Here's how the part is built. I have some questions about the finished solid (model axes, mm). Face numbers are marked on the shaded views. A direction names the side the tool comes from. Round coordinates to 2 decimals unless told otherwise and drop trailing zeros. Loops run counter-clockwise (first coordinate to the right, second up) from the corner with the lowest first, then second, coordinate; pieces in that order, holes last. Notation, with made-up numbers: M -38.5,38 L -31.5,38 A10 cw -31.5,43 Z; hole C 65.25,9.25 d2. An arc over 180 degrees is marked long. Write each question's results on one line, items separated by ' | '. Start each with the question number.
```python
from build123d import *

# Parameters (mm, degrees)
SKETCH1_W           = 40
SKETCH1_H           = 40
BOSS_EXTRUDE1_DEPTH = 10
SKETCH2_R           = 6.5
BOSS_EXTRUDE2_DEPTH = 2
SKETCH3_W           = 7.5
SKETCH3_H           = 20
BOSS_EXTRUDE3_DEPTH = 3
SKETCH4_W           = 6.5
SKETCH4_H           = 1.5
BOSS_EXTRUDE4_DEPTH = 2.5
CUT_EXTRUDE1_DEPTH  = 2.5
CUT_EXTRUDE6_DEPTH  = 12.5
CHAMFER1_SIZE       = 1.5
SKETCH8_W           = 7
SKETCH8_H           = 4
SKETCH8_W_2         = 5
SKETCH8_H_2         = 2
BOSS_EXTRUDE6_DEPTH = 6
SKETCH7_R           = 2.5
SKETCH7_R_2         = 1.5
BOSS_EXTRUDE7_DEPTH = 4.5


with BuildPart() as part:
    # Sketch1 → Boss-Extrude1 (new, symmetric)
    with BuildSketch(Plane.XY):
        Rectangle(SKETCH1_W, SKETCH1_H)
    extrude(amount=BOSS_EXTRUDE1_DEPTH, both=True)

    # Sketch2 → Boss-Extrude2 (add)
    with BuildSketch(Plane(origin=(0, 20, 0), x_dir=(1, 0, 0), z_dir=(0, 1, 0))):
        with Locations(Location((-10, 0, 0), (0, 0, 90))):
            Circle(SKETCH2_R)
    extrude(amount=BOSS_EXTRUDE2_DEPTH)

    # Sketch3 → Boss-Extrude3 (add)
    with BuildSketch(Plane(origin=(0, 7.5, 0), x_dir=(-1, 0, 0), z_dir=(0, -1, 0))):
        with Locations((23.75, 0)):
            Rectangle(SKETCH3_W, SKETCH3_H)
        with Locations((-23.75, 0)):
            Rectangle(SKETCH3_W, SKETCH3_H)
    extrude(amount=-BOSS_EXTRUDE3_DEPTH)

    # Sketch4 → Boss-Extrude4 (add)
    with BuildSketch(Plane(origin=(0, 10.5, 0), x_dir=(1, 0, 0), z_dir=(0, 1, 0))):
        with Locations((23.25, 0)):
            Rectangle(SKETCH4_W, SKETCH4_H)
    boss_extrude4 = extrude(amount=BOSS_EXTRUDE4_DEPTH)

    # Sketch5 → Cut-Extrude1 (cut)
    with BuildSketch(Plane.XY.offset(0.75)):
        Polygon((26.5, 11), (21.5, 13), (26.5, 13), align=None)
    cut_extrude1 = extrude(amount=-CUT_EXTRUDE1_DEPTH, mode=Mode.SUBTRACT)

    # Sketch6 → Cut-Extrude6 (cut)
    with BuildSketch(Plane(origin=(0, 10.5, 0), x_dir=(1, 0, 0), z_dir=(0, 1, 0))):
        with BuildLine():
            Line((-27.449489743, 6.5), (-27.5, 6.5))
            Line((-27.5, 6.5), (-27.5, 5.5))
            Line((-27.5, 5.5), (-27.449489743, 5.5))
            ThreePointArc((-27.449489743, 5.5), (-22.5, 6), (-27.449489743, 6.5))
        make_face()
        with BuildLine():
            Line((-27.449489743, -5.5), (-27.5, -5.5))
            Line((-27.5, -5.5), (-27.5, -6.5))
            Line((-27.5, -6.5), (-27.449489743, -6.5))
            ThreePointArc((-27.449489743, -6.5), (-22.5, -6), (-27.449489743, -5.5))
        make_face()
    cut_extrude6 = extrude(amount=-CUT_EXTRUDE6_DEPTH, mode=Mode.SUBTRACT)

    # Mirror1: Boss-Extrude4, Cut-Extrude1, Cut-Extrude6 across plane
    add(boss_extrude4.mirror(Plane(origin=(0, 0, 0), x_dir=(0, 0, 1), z_dir=(1, 0, 0))))
    add(cut_extrude1.mirror(Plane(origin=(0, 0, 0), x_dir=(0, 0, 1), z_dir=(1, 0, 0))), mode=Mode.SUBTRACT)
    add(cut_extrude6.mirror(Plane(origin=(0, 0, 0), x_dir=(0, 0, 1), z_dir=(1, 0, 0))), mode=Mode.SUBTRACT)

    # Chamfer1
    chamfer1_edges = [part.edges().sort_by_distance(p)[0] for p in [
        (-10, 22, 6.5),
    ]]
    chamfer(chamfer1_edges, length=CHAMFER1_SIZE)

    # Sketch8 → Boss-Extrude6 (add)
    with BuildSketch(Plane.ZY.offset(20)):
        with Locations((0, -11)):
            Rectangle(SKETCH8_W, SKETCH8_H)
        with Locations((0, -11)):
            Rectangle(SKETCH8_W_2, SKETCH8_H_2, mode=Mode.SUBTRACT)
    extrude(amount=BOSS_EXTRUDE6_DEPTH)

    # Sketch7 → Boss-Extrude7 (add)
    with BuildSketch(Plane(origin=(0, 22, 0), x_dir=(1, 0, 0), z_dir=(0, 1, 0))):
        with Locations(Location((-10, 0, 0), (0, 0, 270))):
            Circle(SKETCH7_R)
        with Locations(Location((-10, 0, 0), (0, 0, 270))):
            Circle(SKETCH7_R_2, mode=Mode.SUBTRACT)
    extrude(amount=BOSS_EXTRUDE7_DEPTH)


solid = part.part
```
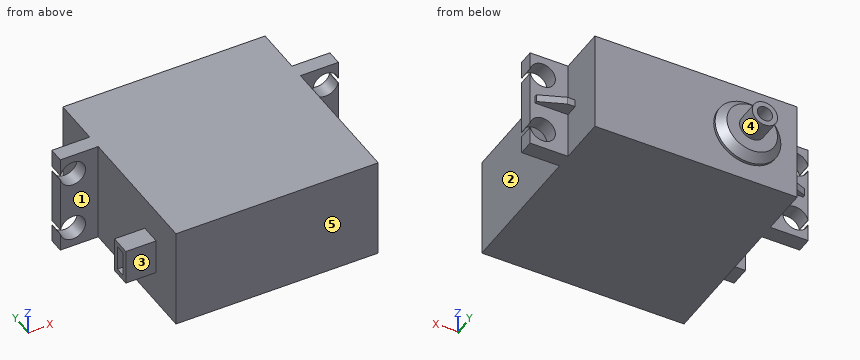
Item 1: I need wall thicknesses on L1, parallel to Z at x = 25, y = 9.3; L2, parallel to Y at x = -19, z = 8; L3, parallel to X at y = 9.9, z = 6. Which ranges of each line are inside material? Lowest first, please.
Item 2: If we section it at A-A on x = -25: Please give me the cut outline in (y, z).
Item 3: If we section it at C-C on y = -11: Please give me the cut outline in (x, z).
Item 4: If we section it at D-D on y = 8.5: Please give me the cut outline in (x, z), and give its area (3 significant figures).
Item 5: I'm going to push flat-ended pins straight in: pin 1 (4.5 mm diameter, centred on x = -22.5, y = -10.5, fed in from -Z); pin 2 (5 mm diameter, centred on x = 11.5, z = -1, fed in from +Y); pin 3 (3 mm diameter, centred on x = -23, z = -1, fed in from +Y); pin 4 (4 mm diameter, centred on x = -25, z = 6, fed in from -Y). Where does each tip first touch, or does it pass through?
Item 6: Which directions (+Z, -Z, +X, -X, +Y, -Y) give clear straight access to the entire face, cutting with the end or side of a thin tool? Please do the marked faces 1, 2, 3, 4 and 5.
Item 7: If we section it at B-B on x = 25: Please give me the cut outline in (y, z), and give its area (4 significant figures).
Numbers:
1) L1: -10 to -8.5, -3.5 to 3.5, 8.5 to 10 | L2: -20 to 20 | L3: -22.5 to 22.5
2) outline: M -13,-3.5 L -9,-3.5 L -9,3.5 L -13,3.5 Z; M 7.5,-10 L 10.5,-10 L 10.5,-8.5 L 7.5,-8.5 Z; M 7.5,-3.5 L 10.5,-3.5 L 10.5,-0.75 L 11.6,-0.75 L 11.6,0.75 L 10.5,0.75 L 10.5,3.5 L 7.5,3.5 Z; M 7.5,8.5 L 10.5,8.5 L 10.5,10 L 7.5,10 Z; hole M -12,-2.5 L -10,-2.5 L -10,2.5 L -12,2.5 Z
3) outline: M -26,-3.5 L -20,-3.5 L -20,-10 L 20,-10 L 20,10 L -20,10 L -20,3.5 L -26,3.5 L -26,2.5 L -20,2.5 L -20,-2.5 L -26,-2.5 Z
4) outline: M -27.5,-10 L 27.5,-10 L 27.5,-6.5 L 27.45,-6.5 A2.5 cw long 27.45,-5.5 L 27.5,-5.5 L 27.5,5.5 L 27.45,5.5 A2.5 cw long 27.45,6.5 L 27.5,6.5 L 27.5,10 L -27.5,10 L -27.5,6.5 L -27.45,6.5 A2.5 cw long -27.45,5.5 L -27.5,5.5 L -27.5,-5.5 L -27.45,-5.5 A2.5 cw long -27.45,-6.5 L -27.5,-6.5 Z | area: 1,020 mm²
5) pin 1: z = -3.5 | pin 2: y = 20 | pin 3: y = 12.99 | pin 4: through
6) face 1: +Z, -Z, -X | face 2: +Z, -Z, +X, -Y | face 3: +Z, -Z, -X, -Y | face 4: +Y | face 5: +Z, -Z, +X, -X, -Y
7) outline: M 7.5,-10 L 10.5,-10 L 10.5,-8.5 L 7.5,-8.5 Z; M 7.5,-3.5 L 10.5,-3.5 L 10.5,-0.75 L 11.6,-0.75 L 11.6,0.75 L 10.5,0.75 L 10.5,3.5 L 7.5,3.5 Z; M 7.5,8.5 L 10.5,8.5 L 10.5,10 L 7.5,10 Z | area: 31.65 mm²
